Model file for the job. Use its own axes, mm. A direction names the side the tool comes from. Round coordinates to 2 decimals unless told otherwise and drop trailing zeros. Loops run counter-clockwise (first coordinate to the right, second up) from the corner with the lowest first, then second, coordinate; pieces in that order, holes last.
from build123d import *

# Parameters (mm, degrees)
SKETCH1_R           = 8
BOSS_EXTRUDE1_DEPTH = 4.1
FILLET1_R           = 0.5
CHAMFER1_START      = 5.365714371
CHAMFER1_OUTLINE_W  = 7
CHAMFER1_OUTLINE_H  = 10
CHAMFER1_DEPTH      = 2.634285629
FILLET2_R           = 1


with BuildPart() as part:
    # Sketch1 → Boss-Extrude1 (new body)
    with BuildSketch(Plane(origin=(0, 0, 0), x_dir=(0, 0, -1), z_dir=(1, 0, 0))):
        with BuildLine():
            Line((-0.008202263, 0.000360071), (-8.869837301, 8.519305154))
            Line((-8.869837301, 8.519305154), (22.061371293, 8.519305154))
            ThreePointArc((22.061371293, 8.519305154), (44.698252536, 4.645550739), (22.061797737, 0.769305154))
            Line((22.061797737, 0.769305154), (6.991797737, 0.769305154))
            Line((6.991797737, 0.769305154), (6.991797737, 5.53817988))
            Line((6.991797737, 5.53817988), (-0.008202263, 5.53817988))
            Line((-0.008202263, 5.53817988), (-0.008202263, 0.000360071))
        make_face()
        with Locations((33.048252553, 4.644909697)):
            Circle(SKETCH1_R, mode=Mode.SUBTRACT)
    extrude(amount=BOSS_EXTRUDE1_DEPTH)

    # Fillet1
    fillet1_edges = [part.edges().sort_by_distance(p)[0] for p in [
        (2.05, 0.000360071, 0.008202263),
    ]]
    fillet(fillet1_edges, radius=FILLET1_R)

    # Chamfer1: read off the stored shape, not the designer's step
    # Chamfer1 outline → Chamfer1 (cut)
    with BuildSketch(Plane(origin=(0, 0, 0), x_dir=(-0.10573160402996473, 0.993935733552454, -0.03020902972284707), z_dir=(0.955693010226633, 0.10996252801543402, 0.273055145779038)).offset(CHAMFER1_START)):
        with Locations((5.5, 4)):
            Rectangle(CHAMFER1_OUTLINE_W, CHAMFER1_OUTLINE_H)
    extrude(amount=CHAMFER1_DEPTH, mode=Mode.SUBTRACT)

    # Fillet2
    fillet2_edges = [part.edges().sort_by_distance(p)[0] for p in [
        (3.1, 8.519305154, 5.369837302),
        (3.1, 6.093699523, 6.346657301),
    ]]
    fillet(fillet2_edges, radius=FILLET2_R)


solid = part.part
Q1. Flat gauge pins, fed straight in: P1, Ø2, axis at x = 1.5, z = -15.5, coming from the -Y side; P2, Ø1.5, axis at x = 2.5, y = 9, coming from the -Z side; P3, Ø2, axis at x = 0.5, z = -3, coming from the +Y side; P4, Ø6, axis at y = 2, z = -35.5, coming from the +X side. Where does each tip first touch, or does it go through?
Q2. Pull direction Y, two halves, no side cores. Call faces 4 (the face through (1.57, 3.76, 3.92)), 5 (the face through (2.838, 8.368, 4.954)), 6 (the face through (2.02, 5.1, -44.69)), 7 (the face through (2.02, 7.05, -40.68)): pulls with the +Y half, pulls with the -Y half, needs draft (parallel to the pull), parting line crosses it, or undercut.
Q3. Slice it at A-A on y = -1. Give the cut face in (x, z).
Q4. Slice it at D-D on z = -13. Give the cut face in (x, y).
Q5. Slice it at B-B on z = -34. Give the cut face in (x, y), plus the area to 3 significant figures.
Q6. Probe line 1 (Z direction, x = 2.65, y = 3); line 2 (Y direction, x = 3.75, z = -6.5); line 3 (Z direction, x = 1, y = 12). List the from-to ranges inside material, lowest first.
Q7. Slice it at C-C on x = 0.6. Give the cut face in (y, z), plus the area to 3 significant figures.
Q8. Tool access for faces 1 (the face through (2, 5.538, -4)), 2 (the face through (2, 8.519, -6)), 3 (the face through (4.1, 5, -24)): list every direction of +Z, -Z, +X, -X, +Y, -Y with a clear straight run to the whole face (end or side of a thin tool).
Reply:
1. P1: stops at y = 0.77
1. P2: stops at z = -44.13
1. P3: stops at y = 8.52
1. P4: passes through
2. face 4: pulls with the -Y half
2. face 5: pulls with the +Y half
2. face 6: parting line crosses it
2. face 7: undercut
3. outline: (0, -43.24) - (4.1, -43.24) - (4.1, -38.72) - (0, -38.72) - close; (0, -27.38) - (4.1, -27.38) - (4.1, -22.86) - (0, -22.86) - close
4. outline: (0, 0.77) - (4.1, 0.77) - (4.1, 8.52) - (0, 8.52) - close
5. outline: (0, -6.97) - (4.1, -6.97) - (4.1, -3.3) - (0, -3.3) - close; (0, 12.59) - (4.1, 12.59) - (4.1, 16.26) - (0, 16.26) - close
5. area: 30.1 mm2
6. line 1: z = -44.58 to -40.88, -25.22 to -6.99, 0.01 to 3.13
6. line 2: y = 5.54 to 8.52
6. line 3: z = -42.08 to -36.2, -29.9 to -24.01
7. outline: (0.77, -22.06) arc R11.65 ccw (long way) to (8.52, -22.06) - (8.52, 8.87) - (0.81, 0.85) arc R0.5 ccw to (1.17, 0.01) - (5.54, 0.01) - (5.54, -6.99) - (0.77, -6.99) - close; hole circle Ø16 at (4.64, -33.05)
7. area: 397 mm2
8. face 1: +X, -X, -Y
8. face 2: +Z, +X, -X, +Y
8. face 3: +Z, -Z, +X, +Y, -Y
